Geometry check sheet. Reference: the model listing, model coordinates, mm. A direction names the side the tool comes from. Coordinates: 2 decimals unless noted, no trailing zeros. Loops run counter-clockwise (first coordinate to the right, second up) from the corner with the lowest first, then second, coordinate; pieces in that order, holes last.
from build123d import *

# Parameters (mm, degrees)
BOSS_EXTRUDE1_DEPTH = 3
SKETCH2_R           = 1.6
CUT_EXTRUDE1_DEPTH  = 64.710281745
MOVE_FACE1_BY       = 0.5
MOVE_FACE1_2_BY     = 0.5
MOVE_FACE1_3_BY     = 0.5
MOVE_FACE1_4_BY     = 0.5
MOVE_FACE1_5_BY     = 0.5
MOVE_FACE1_6_BY     = 0.5
MOVE_FACE1_7_BY     = 0.5
MOVE_FACE1_8_BY     = 0.5
MOVE_FACE1_9_BY     = 0.5
MOVE_FACE1_10_BY    = 0.5
BOSS_EXTRUDE2_DEPTH = 1
FILLET1_R           = 0.5
CUT_EXTRUDE2_DEPTH  = 64.003968129
FILLET2_R           = 1


with BuildPart() as part:
    # Sketch1 → Boss-Extrude1 (new body)
    with BuildSketch(Plane.XY):
        with BuildLine():
            Line((16.464466094, 43.535533906), (43.535533906, 16.464466094))
            ThreePointArc((43.535533906, 16.464466094), (44.619397663, 14.84234935), (45, 12.928932188))
            Line((45, 12.928932188), (45, 5))
            ThreePointArc((45, 5), (43.535533906, 1.464466094), (40, 0))
            Line((40, 0), (5, 0))
            ThreePointArc((5, 0), (1.464466094, 1.464466094), (0, 5))
            Line((0, 5), (0, 40))
            ThreePointArc((0, 40), (1.464466094, 43.535533906), (5, 45))
            Line((5, 45), (12.928932188, 45))
            ThreePointArc((12.928932188, 45), (14.84234935, 44.619397663), (16.464466094, 43.535533906))
        make_face()
    extrude(amount=BOSS_EXTRUDE1_DEPTH)

    # Sketch2 → Cut-Extrude1 (cut, through all)
    with BuildSketch(Plane.XY.offset(3)):
        with Locations((7.5, 37.5)):
            Circle(SKETCH2_R)
        with Locations((7.5, 22.5)):
            Circle(SKETCH2_R)
        with Locations((22.5, 7.5)):
            Circle(SKETCH2_R)
        with Locations((37.5, 7.5)):
            Circle(SKETCH2_R)
    extrude(amount=-CUT_EXTRUDE1_DEPTH, mode=Mode.SUBTRACT)

    # Move Face1: a curved face moved inward by 0.5
    add(Solid.thicken(part.faces().sort_by_distance((1.464466094, 1.464466094, 1.5))[0], -MOVE_FACE1_BY), mode=Mode.SUBTRACT)

    # Move Face1 2: a face moved inward by 0.5
    extrude(part.faces().sort_by_distance((22.5, 0, 1.5))[0], amount=MOVE_FACE1_2_BY, dir=(0, 1, 0), mode=Mode.SUBTRACT)

    # Move Face1 3: a curved face moved inward by 0.5
    add(Solid.thicken(part.faces().sort_by_distance((43.535533906, 1.464466094, 1.5))[0], -MOVE_FACE1_3_BY), mode=Mode.SUBTRACT)

    # Move Face1 4: a face moved inward by 0.5
    extrude(part.faces().sort_by_distance((45, 8.964466094, 1.5))[0], amount=MOVE_FACE1_4_BY, dir=(-1, 0, 0), mode=Mode.SUBTRACT)

    # Move Face1 5: a curved face moved inward by 0.5
    add(Solid.thicken(part.faces().sort_by_distance((44.619397663, 14.84234935, 1.5))[0], -MOVE_FACE1_5_BY), mode=Mode.SUBTRACT)

    # Move Face1 6: a face moved inward by 0.5
    extrude(part.faces().sort_by_distance((30, 30, 1.5))[0], amount=MOVE_FACE1_6_BY, dir=(-0.707106781, -0.707106781, 0), mode=Mode.SUBTRACT)

    # Move Face1 7: a curved face moved inward by 0.5
    add(Solid.thicken(part.faces().sort_by_distance((14.84234935, 44.619397663, 1.5))[0], -MOVE_FACE1_7_BY), mode=Mode.SUBTRACT)

    # Move Face1 8: a face moved inward by 0.5
    extrude(part.faces().sort_by_distance((8.964466094, 45, 1.5))[0], amount=MOVE_FACE1_8_BY, dir=(0, -1, 0), mode=Mode.SUBTRACT)

    # Move Face1 9: a curved face moved inward by 0.5
    add(Solid.thicken(part.faces().sort_by_distance((1.464466094, 43.535533906, 1.5))[0], -MOVE_FACE1_9_BY), mode=Mode.SUBTRACT)

    # Move Face1 10: a face moved inward by 0.5
    extrude(part.faces().sort_by_distance((0, 22.5, 1.5))[0], amount=MOVE_FACE1_10_BY, dir=(1, 0, 0), mode=Mode.SUBTRACT)

    # Sketch3 → Boss-Extrude2 (add)
    with BuildSketch(Plane.XY.offset(3)):
        with BuildLine():
            Line((5, 0.5), (40, 0.5))
            ThreePointArc((40, 0.5), (43.181980515, 1.818019485), (44.5, 5))
            Line((44.5, 5), (44.5, 12.928932188))
            ThreePointArc((44.5, 12.928932188), (44.157457896, 14.651007634), (43.181980515, 16.110912703))
            Line((43.181980515, 16.110912703), (16.110912703, 43.181980515))
            ThreePointArc((16.110912703, 43.181980515), (14.651007634, 44.157457896), (12.928932188, 44.5))
            Line((12.928932188, 44.5), (5, 44.5))
            ThreePointArc((5, 44.5), (1.818019485, 43.181980515), (0.5, 40))
            Line((0.5, 40), (0.5, 5))
            ThreePointArc((0.5, 5), (1.818019485, 1.818019485), (5, 0.5))
        make_face()
        with BuildLine():
            Line((5, 2), (40, 2))
            ThreePointArc((40, 2), (42.121320344, 2.878679656), (43, 5))
            Line((43, 5), (43, 12.928932188))
            ThreePointArc((43, 12.928932188), (42.771638598, 14.076982485), (42.121320344, 15.050252532))
            Line((42.121320344, 15.050252532), (15.050252532, 42.121320344))
            ThreePointArc((15.050252532, 42.121320344), (14.076982485, 42.771638598), (12.928932188, 43))
            Line((12.928932188, 43), (5, 43))
            ThreePointArc((5, 43), (2.878679656, 42.121320344), (2, 40))
            Line((2, 40), (2, 5))
            ThreePointArc((2, 5), (2.878679656, 2.878679656), (5, 2))
        make_face(mode=Mode.SUBTRACT)
    extrude(amount=BOSS_EXTRUDE2_DEPTH)

    # Fillet1
    fillet1_edges = [part.edges().sort_by_distance(p)[0] for p in [
        (1.818019485, 1.818019485, 4),
        (22.5, 0.5, 4),
        (43.181980515, 1.818019485, 4),
        (44.5, 8.964466094, 4),
        (44.157457896, 14.651007634, 4),
        (29.646446609, 29.646446609, 4),
        (14.651007634, 44.157457896, 4),
        (8.964466094, 44.5, 4),
        (1.818019485, 43.181980515, 4),
        (0.5, 22.5, 4),
        (2.878679656, 2.878679656, 4),
        (22.5, 2, 4),
        (42.121320344, 2.878679656, 4),
        (43, 8.964466094, 4),
        (42.771638598, 14.076982485, 4),
        (28.585786438, 28.585786438, 4),
        (14.076982485, 42.771638598, 4),
        (8.964466094, 43, 4),
        (2.878679656, 42.121320344, 4),
        (2, 22.5, 4),
    ]]
    fillet(fillet1_edges, radius=FILLET1_R)

    # Sketch4 → Cut-Extrude2 (cut, through all)
    with BuildSketch(Plane.XY.offset(3)):
        with BuildLine():
            Line((15.5, 27.650757595), (15.5, 17.5))
            ThreePointArc((15.5, 17.5), (16.085786438, 16.085786438), (17.5, 15.5))
            Line((17.5, 15.5), (27.650757595, 15.5))
            ThreePointArc((27.650757595, 15.5), (29.49851666, 16.734633135), (29.064971157, 18.914213562))
            Line((29.064971157, 18.914213562), (18.914213562, 29.064971157))
            ThreePointArc((18.914213562, 29.064971157), (16.734633135, 29.49851666), (15.5, 27.650757595))
        make_face()
    extrude(amount=-CUT_EXTRUDE2_DEPTH, mode=Mode.SUBTRACT)

    # Fillet2
    fillet2_edges = [part.edges().sort_by_distance(p)[0] for p in [
        (16.085786438, 16.085786438, 3),
        (22.575378798, 15.5, 3),
        (29.49851666, 16.734633135, 3),
        (23.98959236, 23.98959236, 3),
        (16.734633135, 29.49851666, 3),
        (15.5, 22.575378798, 3),
    ]]
    fillet(fillet2_edges, radius=FILLET2_R)


solid = part.part
(1) Sectioned sample at A-A on x = 7.5. Record the cut outline in (y, z).
Findings:
outline: (0.5, 0) - (20.9, 0) - (20.9, 3) - (2, 3) - (2, 3.5) arc R0.5 ccw to (1.5, 4) - (1, 4) arc R0.5 ccw to (0.5, 3.5) - close; (24.1, 0) - (35.9, 0) - (35.9, 3) - (24.1, 3) - close; (39.1, 0) - (44.5, 0) - (44.5, 3.5) arc R0.5 ccw to (44, 4) - (43.5, 4) arc R0.5 ccw to (43, 3.5) - (43, 3) - (39.1, 3) - close
(2) Access from +Z, -Z, +X, -X, +Y, -Y to the whole of each face (thin tool, end or side, straight path). Record for faces 4 (the flat face through (23, 15.5, 1)), 5 (the flat face through (22, 0.5, 2)), 6 (the cylindrical face through (2.9, 42.14, 3.25)).
Findings:
face 4: +Z, -Z
face 5: +Z, -Z, +X, -X, -Y
face 6: +Z
(3) Scan lines: L1, parallel to Y at x = 7.5, z = 0.65; L2, parallel to Z at x = 17, y = 4; L3, parallel to X at y = 16.5, z = 3.85. Record each from-to range of solid material in increasing order.
Findings:
L1: y = 0.5 to 20.9, 24.1 to 35.9, 39.1 to 44.5
L2: z = 0 to 3
L3: x = 0.64 to 1.86, 40.87 to 42.59
(4) Gauge pin test, flat ends, axial feed: pin 1 Ø2 at (y, z) = (14.5, 3) entering from +X; pin 2 Ø3 at (x, y) = (22.5, 7.5) entering from -Z; pin 3 Ø2 at (y, z) = (20, 1) entering from +X; pin 4 Ø8 at (x, y) = (25.5, 7) entering from +Z. Record the tip position at first contact, or that the pin passes through.
Findings:
pin 1: stops at x = 44.46
pin 2: passes through
pin 3: stops at x = 40.29
pin 4: stops at z = 3
(5) Draft check along X on faces 1 (the flat face through (9, 44.5, 2)), 2 (the flat face through (28.775, 28.396, 3.246)), 3 (the cylindrical face through (29.356, 29.735, 3.85)). Enter one of: +X half, -X half, draft (parallel to the pull), parting line (faces both ways), or undercut.
Findings:
face 1: draft
face 2: undercut
face 3: +X half
(6) Sectioned sample at C-C on z = 1.25. Record the cut outline in (x, y), and give its area (3 significant figures).
Findings:
outline: (0.5, 5) arc R4.5 ccw to (5, 0.5) - (40, 0.5) arc R4.5 ccw to (44.5, 5) - (44.5, 12.93) arc R4.5 ccw to (43.18, 16.11) - (16.11, 43.18) arc R4.5 ccw to (12.93, 44.5) - (5, 44.5) arc R4.5 ccw to (0.5, 40) - close; hole circle Ø3.2 at (7.5, 22.5); hole circle Ø3.2 at (7.5, 37.5); hole (15.5, 17.5) arc R2 ccw to (17.5, 15.5) - (27.65, 15.5) arc R2 ccw to (29.06, 18.91) - (18.91, 29.06) arc R2 ccw to (15.5, 27.65) - close; hole circle Ø3.2 at (22.5, 7.5); hole circle Ø3.2 at (37.5, 7.5)
area: 1,320 mm2
(7) Sectioned sample at D-D on y = 12. Record the cut outline in (x, z), and give its area (3 significant figures).
Findings:
outline: (0.5, 0) - (44.5, 0) - (44.5, 3.5) arc R0.5 ccw to (44, 4) - (43.5, 4) arc R0.5 ccw to (43, 3.5) - (43, 3) - (2, 3) - (2, 3.5) arc R0.5 ccw to (1.5, 4) - (1, 4) arc R0.5 ccw to (0.5, 3.5) - close
area: 135 mm2
